Part model, mm, in its own coordinate system. A direction names the side the tool comes from. Round coordinates to 2 decimals unless told otherwise and drop trailing zeros. Loops run counter-clockwise (first coordinate to the right, second up) from the corner with the lowest first, then second, coordinate; pieces in that order, holes last.
(1) Cut at A-A on x = 0. List the corners of the cut face in (y, z).
(2) Cut at D-D on y = -7.75. List the corners of the cut face in (x, z), then the cut area to 3 significant figures.
(3) Cut at C-C on z = -7.75. List the corners of the cut face in (x, y).
(4) Cut at B-B on y = 0. List the corners of the cut face in (x, z).
(5) Tool access for faces 1 (the face through (18.25, 10, -9)), 2 (the face through (18.25, 0, -2)), 3 (the face through (-16.75, -0.2, -13.4)), 4 (the face through (-19, 9.75, -8)): list every direction of +Z, -Z, +X, -X, +Y, -Y with a clear straight run to the whole face (end or side of a thin tool).
(6) Probe probe 1 along Y at (x, z) = (-14.75, -2.2); probe 2 along X at (y, z) = (-7.25, -15.25); probe 3 along Y at (x, z) = (0, -0.6). List the from-to ranges inside material, lowest first.
(7) Mould opens along Y. For faces 5 (the face through (18, 0, -13)), 6 (the face through (16.75, -0.2, -13.4)) say: +Y half, -Y half, draft (parallel to the pull), parting line (faces both ways), or undercut.
(8) Flat gauge pins, fed straight in: pin 1 (3 mm diameter, centred on x = 13.5, z = -11.5, fed in from +Y); pin 2 (0.8 mm diameter, centred on x = -17.5, y = -2.5, fed in from +Z); pin 3 (8 mm diameter, centred on y = 0, z = -3, fed in from +X); pin 4 (4.5 mm diameter, centred on y = 4, z = -2.5, fed in from -X). Where does each tip first touch, or does it go through?
from build123d import *

# Parameters (mm, degrees)
SKETCH2_W           = 36.5
SKETCH2_H           = 27.5
SKETCH2_R           = 11.5
SKETCH2_R_2         = 1.3
BOSS_EXTRUDE1_DEPTH = 1
SKETCH4_R           = 1.3
BOSS_EXTRUDE2_DEPTH = 3
SKETCH5_W           = 1.5
SKETCH5_H           = 27.5
BOSS_EXTRUDE3_DEPTH = 12
SKETCH6_W           = 9
SKETCH6_H           = 21.5
CUT_EXTRUDE1_DEPTH  = 1.5
BOSS_EXTRUDE4_REACH = 29.895
SKETCH7_W           = 2
SKETCH7_H           = 4


with BuildPart() as part:
    # Sketch2 → Boss-Extrude1 (new body)
    with BuildSketch(Plane.XY):
        Rectangle(SKETCH2_W, SKETCH2_H)
        Circle(SKETCH2_R, mode=Mode.SUBTRACT)
        with Locations((-14.75, 0)):
            Circle(SKETCH2_R_2, mode=Mode.SUBTRACT)
        with Locations((14.75, 0)):
            Circle(SKETCH2_R_2, mode=Mode.SUBTRACT)
    extrude(amount=-BOSS_EXTRUDE1_DEPTH)

    # Sketch4 → Boss-Extrude2 (add)
    with BuildSketch(Plane(origin=(0, 0, -1), x_dir=(-1, 0, 0), z_dir=(0, 0, -1))):
        with BuildLine():
            Line((-16.75, 4), (-16.75, 13.75))
            Line((-16.75, 13.75), (-18.25, 13.75))
            Line((-18.25, 13.75), (-18.25, -13.75))
            Line((-18.25, -13.75), (-16.75, -13.75))
            Line((-16.75, -13.75), (-16.75, -4))
            ThreePointArc((-16.75, -4), (-16.164213562, -2.585786438), (-14.75, -2))
            ThreePointArc((-14.75, -2), (-12.75, 0), (-14.75, 2))
            ThreePointArc((-14.75, 2), (-16.164213562, 2.585786438), (-16.75, 4))
        make_face()
        with Locations((-14.75, 0)):
            Circle(SKETCH4_R, mode=Mode.SUBTRACT)
    boss_extrude2 = extrude(amount=BOSS_EXTRUDE2_DEPTH)

    # Sketch5 → Boss-Extrude3 (add)
    with BuildSketch(Plane(origin=(0, 0, -4), x_dir=(-1, 0, 0), z_dir=(0, 0, -1))):
        with Locations((-17.5, 0)):
            Rectangle(SKETCH5_W, SKETCH5_H)
    boss_extrude3 = extrude(amount=BOSS_EXTRUDE3_DEPTH)

    # Sketch6 → Cut-Extrude1 (cut)
    with BuildSketch(Plane(origin=(18.25, 0, 0), x_dir=(0, 0, -1), z_dir=(1, 0, 0))):
        with Locations((8.5, 0)):
            Rectangle(SKETCH6_W, SKETCH6_H)
    cut_extrude1 = extrude(amount=-CUT_EXTRUDE1_DEPTH, mode=Mode.SUBTRACT)

    # Boss-Extrude4: up to this face of the body (flat: up to its plane)
    boss_extrude4_end = Plane(part.part.faces().sort_by_distance((-17.792998906, 0, 0))[0])
    # Sketch7 → Boss-Extrude4 (add, up to the picked face)
    with BuildSketch(Plane(origin=(0, 0, -16), x_dir=(-1, 0, 0), z_dir=(0, 0, -1)), mode=Mode.PRIVATE) as boss_extrude4_sk1:
        with Locations((-19.25, 11.75)):
            Rectangle(SKETCH7_W, SKETCH7_H)
    boss_extrude4_tool1 = split(extrude(boss_extrude4_sk1.sketch, amount=-BOSS_EXTRUDE4_REACH, mode=Mode.PRIVATE), bisect_by=boss_extrude4_end, keep=Keep.BOTH, mode=Mode.PRIVATE)
    # Sketch7 → Boss-Extrude4 (add, up to the picked face)
    with BuildSketch(Plane(origin=(0, 0, -16), x_dir=(-1, 0, 0), z_dir=(0, 0, -1)), mode=Mode.PRIVATE) as boss_extrude4_sk2:
        with Locations((-19.25, -11.75)):
            Rectangle(SKETCH7_W, SKETCH7_H)
    boss_extrude4_tool2 = split(extrude(boss_extrude4_sk2.sketch, amount=-BOSS_EXTRUDE4_REACH, mode=Mode.PRIVATE), bisect_by=boss_extrude4_end, keep=Keep.BOTH, mode=Mode.PRIVATE)
    boss_extrude4_1 = boss_extrude4_tool1.solids().sort_by(Axis((19.25, 11.75, -16), (0, 0, 1)))[0]
    add(boss_extrude4_1)
    boss_extrude4_2 = boss_extrude4_tool2.solids().sort_by(Axis((19.25, -11.75, -16), (0, 0, 1)))[0]
    add(boss_extrude4_2)
    boss_extrude4 = boss_extrude4_1 + boss_extrude4_2  # Boss-Extrude4 as one shape, for the pattern or mirror that repeats it

    # Mirror1: Boss-Extrude2, Boss-Extrude3, Cut-Extrude1, Boss-Extrude4 across plane
    add(boss_extrude2.mirror(Plane(origin=(0, 0, 0), x_dir=(0, 0, 1), z_dir=(1, 0, 0))))
    add(boss_extrude3.mirror(Plane(origin=(0, 0, 0), x_dir=(0, 0, 1), z_dir=(1, 0, 0))))
    add(cut_extrude1.mirror(Plane(origin=(0, 0, 0), x_dir=(0, 0, 1), z_dir=(1, 0, 0))), mode=Mode.SUBTRACT)
    add(boss_extrude4.mirror(Plane(origin=(0, 0, 0), x_dir=(0, 0, 1), z_dir=(1, 0, 0))))


solid = part.part
Final values:
1. outline: (-13.75, -1) - (-11.5, -1) - (-11.5, 0) - (-13.75, 0) - close; (11.5, -1) - (13.75, -1) - (13.75, 0) - (11.5, 0) - close
2. outline: (-18.25, -16) - (-16.75, -16) - (-16.75, -13) - (-18.25, -13) - close; (-18.25, -4) - (-16.75, -4) - (-16.75, -1) - (-8.5, -1) - (-8.5, 0) - (-18.25, 0) - close; (8.5, -1) - (16.75, -1) - (16.75, -4) - (18.25, -4) - (18.25, 0) - (8.5, 0) - close; (16.75, -16) - (18.25, -16) - (18.25, -13) - (16.75, -13) - close
2. area: 37.5 mm2
3. outline: (-20.25, -13.75) - (-16.75, -13.75) - (-16.75, -10.75) - (-18.25, -10.75) - (-18.25, -9.75) - (-20.25, -9.75) - close; (-20.25, 9.75) - (-18.25, 9.75) - (-18.25, 10.75) - (-16.75, 10.75) - (-16.75, 13.75) - (-20.25, 13.75) - close; (16.75, -13.75) - (20.25, -13.75) - (20.25, -9.75) - (18.25, -9.75) - (18.25, -10.75) - (16.75, -10.75) - close; (16.75, 10.75) - (18.25, 10.75) - (18.25, 9.75) - (20.25, 9.75) - (20.25, 13.75) - (16.75, 13.75) - close
4. outline: (-18.25, -16) - (-16.75, -16) - (-16.75, -13) - (-18.25, -13) - close; (-18.25, -4) - (-16.05, -4) - (-16.05, 0) - (-18.25, 0) - close; (-13.45, -4) - (-12.75, -4) - (-12.75, -1) - (-11.5, -1) - (-11.5, 0) - (-13.45, 0) - close; (11.5, -1) - (12.75, -1) - (12.75, -4) - (13.45, -4) - (13.45, 0) - (11.5, 0) - close; (16.05, -4) - (18.25, -4) - (18.25, 0) - (16.05, 0) - close; (16.75, -16) - (18.25, -16) - (18.25, -13) - (16.75, -13) - close
5. face 1: none
5. face 2: +Z, -Z, +X
5. face 3: -Z
5. face 4: +Z, -Z, -X
6. probe 1: y = -2 to -1.3, 1.3 to 2
6. probe 2: x = -18.25 to -16.75, 16.75 to 18.25
6. probe 3: y = -13.75 to -11.5, 11.5 to 13.75
7. face 5: undercut
7. face 6: draft
8. pin 1: passes through
8. pin 2: stops at z = 0
8. pin 3: stops at x = 18.25
8. pin 4: stops at x = -18.25
